Geometry: final body of the model. Coordinates: model frame, mm. A direction names the side the tool comes from. Round coordinates to 2 decimals unless told otherwise and drop trailing zeros. Write each loop counter-clockwise with the first axis right and the second up, starting at its lowest first coordinate (ties: lowest second). Pieces come first, ordered by that corner, then holes.
from build123d import *

# Parameters (mm, degrees)
F1_DEPTH = 63.5
F0_W     = 25.4
F0_H     = 19.05
F2_DEPTH = 25.4
F3_DEPTH = 7.9375
F5_R     = 6.35


with BuildPart() as f1:
    # F0 (on Front) → F1 (new body, symmetric)
    with BuildSketch(Plane.XZ):
        Polygon((41.275, -9.525), (41.275, 9.525), (22.225, 9.525), (-41.275, 9.525), (-41.275, -9.525), align=None)
    extrude(amount=F1_DEPTH, both=True)

    # F0 (on Front) → F2 (join, symmetric)
    with BuildSketch(Plane.XZ):
        with BuildLine():
            Line((22.225, 9.525), (41.275, 9.525))
            Line((41.275, 9.525), (41.275, 27.0002))
            ThreePointArc((41.275, 27.0002), (45.9246798487, 38.2255201513), (57.15, 42.8752))
            Line((57.15, 42.8752), (66.675, 42.8752))
            Line((66.675, 42.8752), (66.675, 61.9252))
            Line((66.675, 61.9252), (57.15, 61.9252))
            add(Edge.make_bspline(
                [(56.9028538387, 61.9243255263), (56.9851686946, 61.9246577884), (57.0675507307, 61.9249493028), (57.15, 61.9252)],
                knots=[111.3887853631, 111.3887853631, 111.3887853631, 111.3887853631, 111.5045361635, 111.5045361635, 111.5045361635, 111.5045361635], degree=3))
            ThreePointArc((56.9028538387, 61.9243255263), (32.3670703438, 51.6083698356), (22.225, 27.0002))
            Line((22.225, 27.0002), (22.225, 9.525))
        make_face()
        with Locations((79.375, 52.4002)):
            Rectangle(F0_W, F0_H)
    extrude(amount=F2_DEPTH, both=True)

    # F0 (on Front) → F3 (join, symmetric)
    with BuildSketch(Plane.XZ):
        Polygon((41.275, -9.525), (41.275, 9.525), (22.225, 9.525), (-41.275, 9.525), (-41.275, -9.525), align=None)
        with BuildLine():
            Line((22.225, 9.525), (41.275, 9.525))
            Line((41.275, 9.525), (41.275, 27.0002))
            ThreePointArc((41.275, 27.0002), (45.9246798487, 38.2255201513), (57.15, 42.8752))
            Line((57.15, 42.8752), (66.675, 42.8752))
            Line((66.675, 42.8752), (66.675, 61.9252))
            Line((66.675, 61.9252), (57.15, 61.9252))
            add(Edge.make_bspline(
                [(56.9028538387, 61.9243255263), (56.9851686946, 61.9246577884), (57.0675507307, 61.9249493028), (57.15, 61.9252)],
                knots=[111.3887853631, 111.3887853631, 111.3887853631, 111.3887853631, 111.5045361635, 111.5045361635, 111.5045361635, 111.5045361635], degree=3))
            ThreePointArc((56.9028538387, 61.9243255263), (32.3670703438, 51.6083698356), (22.225, 27.0002))
            Line((22.225, 27.0002), (22.225, 9.525))
        make_face()
        with Locations((79.375, 52.4002)):
            Rectangle(F0_W, F0_H)
        with BuildLine():
            Line((-41.275, 9.525), (22.225, 9.525))
            Line((22.225, 9.525), (22.225, 27.0002))
            ThreePointArc((22.225, 27.0002), (32.3670703438, 51.6083698356), (56.9028538387, 61.9243255263))
            add(Edge.make_bspline(
                [(-41.275, 9.525), (-39.3105568509, 23.5502866189), (-22.3100050541, 61.6045845118), (56.9028538387, 61.9243255263)],
                knots=[0, 0, 0, 0, 111.3887853631, 111.3887853631, 111.3887853631, 111.3887853631], degree=3))
        make_face()
    extrude(amount=F3_DEPTH, both=True)

    # F0 (on Front) → F4 (revolve)
    with BuildSketch(Plane.XZ):
        Polygon((92.075, 61.9252), (92.075, 42.8752), (92.075, 38.1), (117.475, 38.1), (117.475, 66.675), (92.075, 66.675), align=None)
    revolve(axis=Axis((92.075, 0, 52.3875), (0, 0, 1)))

    # F5
    f5_edges = [f1.edges().sort_by_distance(p)[0] for p in [
        (-41.275, -63.5, 0),
        (41.275, -63.5, 0),
        (41.275, 63.5, 0),
        (-41.275, 63.5, 0),
    ]]
    fillet(f5_edges, radius=F5_R)


solid = f1.part
1) Section A-A on x = 76. Output: boundary loops of the cut face in (y, z) (3 decimals), plus the area to 3 significant figures.
2) First-contact query: P1, Ø5, axis at y = -16.5, z = 15, coming from the -X side (3 decimals); P2, Ø15.5, axis at x = 29.5, z = 32.5, coming from the -Y side; P3, Ø16.5, axis at x = 1, y = -43, coming from the +Z side (3 decimals). Flat tips, straight axial feed; report the tip coordinate or a pass-through.
3) Section B-B on y = -30. Output: boundary loops of the cut face in (x, z) (3 decimals), plus the area to 3 significant figures.
4) Reachability of faces 1 (the flat face through (49, 25.4, 42)), 2 (the cylindrical face through (45.8, -0.4, 38.1)), 3 (the flat face through (-4, 7.938, 30)), 4 (the flat face through (41.275, -1, 4)) from +Z, -Z, +X, -X, +Y, -Y: full face, straight path, thin tool, end or side. Return the list, or none.
5) Draft query along X for faces 5 (the cylindrical face through (-39.365, -61.689, -0.133)), 6 (the flat face through (63, 0, 42.875)), 7 (the flat face through (49, -25.4, 42)). Return one class per face: pulls with the +X half, pulls with the -X half, needs draft (parallel to the pull), parting line crosses it, or undercut.
6) Line query: probe 1 along Y at (x, z) = (-5, 29); probe 2 along Z at (x, y) = (84, 22) (3 decimals); probe 3 along Z at (x, y) = (7, -14.5) (3 decimals). Output: solid intervals per line, ascending.
Filled in:
1. outline: (-25.4, 42.875) - (-19.666, 42.875) - (-19.666, 38.1) - (19.666, 38.1) - (19.666, 42.875) - (25.4, 42.875) - (25.4, 61.925) - (19.666, 61.925) - (19.666, 66.675) - (-19.666, 66.675) - (-19.666, 61.925) - (-25.4, 61.925) - close
1. area: 1,340 mm2
2. P1: stops at x = 22.225
2. P2: stops at y = -25.4
2. P3: stops at z = 9.525
3. outline: (-41.275, -9.525) - (41.275, -9.525) - (41.275, 9.525) - (-41.275, 9.525) - close
3. area: 1,570 mm2
4. face 1: +Z, +X, -X, +Y
4. face 2: -Z, +Y, -Y
4. face 3: +Z, -X, +Y
4. face 4: -Z, +X, +Y, -Y
5. face 5: pulls with the -X half
5. face 6: undercut
5. face 7: needs draft
6. probe 1: y = -7.94 to 7.94
6. probe 2: z = 38.1 to 66.675
6. probe 3: z = -9.525 to 9.525
